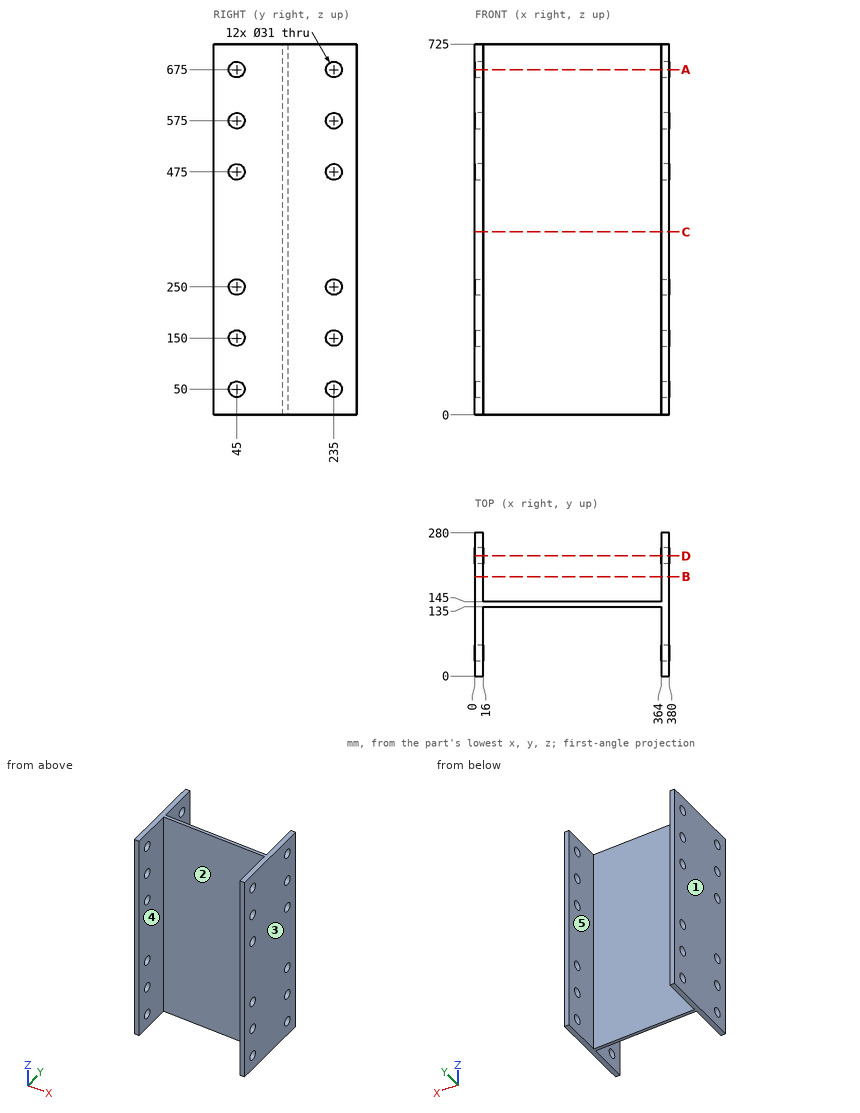
Here's the drawing with two shaded views (mm, measured from the low corner). I have some questions. A direction names the side the tool comes from. Give positions to 0.01 mm unless a question says otherwise; leave off trailing zeros. Loops run counter-clockwise (first coordinate to the right, second up) from the corner with the lowest first, then second, coordinate; pieces in that order, holes last. Notation, with made-up numbers: M 60.25,-5 L 94.25,-5 A16 ccw 94.25,7 Z; hole C -21.75,54 d5. An arc over 180 degrees is marked long. Use one line per item in the form item = value. Start each with the question number.
(1) I want a section at B-B, the plane y = 194.5. Write out the boundary of the cut face in (x, z), and give its area (3 significant figures).
(2) Thinking about a two-plate mould opening in X: for the marked faces 1, 2 and 3, which applies, released by +X, released by -X, zero draft, split by the parting line, or undercut?
(3) I want a section at A-A, the plane z = 675. Write out the boundary of the cut face in (x, y).
(4) I want a section at D-D, the plane y = 235. State how many separate pieces and enclosed holes the cut face has, and give its area (3 significant figures).
(5) On a 3-axis mill with a long thin cutter (end or side, diameter ignored), from which of +Z, -Z, +X, -X, +Y, -Y can I reach the whole of each face in a straight line? I mean the marked faces 4 and 5. Say none if no direction works.
(6) I want a section at C-C, the plane z = 357.5. Write out the boundary of the cut face in (x, y).
(7) Please list where these lines run through material, in increasing order: line 1 (Y direction, x = 371.5, z = 150); line 2 (X direction, y = 164, z = 183.5); line 3 (Y direction, x = 96, z = 276).
Worked out:
q1.outline = M 0,0 L 16,0 L 16,725 L 0,725 Z; M 364,0 L 380,0 L 380,725 L 364,725 Z
q1.area = 23,200 mm²
q2.face_1 = released by -X
q2.face_2 = undercut
q2.face_3 = released by +X
q3.outline = M 0,0 L 16,0 L 16,29.5 L 0,29.5 Z; M 0,60.5 L 16,60.5 L 16,135 L 364,135 L 364,60.5 L 380,60.5 L 380,219.5 L 364,219.5 L 364,145 L 16,145 L 16,219.5 L 0,219.5 Z; M 0,250.5 L 16,250.5 L 16,280 L 0,280 Z; M 364,0 L 380,0 L 380,29.5 L 364,29.5 Z; M 364,250.5 L 380,250.5 L 380,280 L 364,280 Z
q4.separate_pieces = 14
q4.enclosed_holes = 0
q4.area = 17,200 mm²
q5.face_4 = +Z, -Z, -Y
q5.face_5 = +Z, -Z, +Y
q6.outline = M 0,0 L 16,0 L 16,135 L 364,135 L 364,0 L 380,0 L 380,280 L 364,280 L 364,145 L 16,145 L 16,280 L 0,280 Z
q7.line_1 = 0 to 29.5, 60.5 to 219.5, 250.5 to 280
q7.line_2 = 0 to 16, 364 to 380
q7.line_3 = 135 to 145
